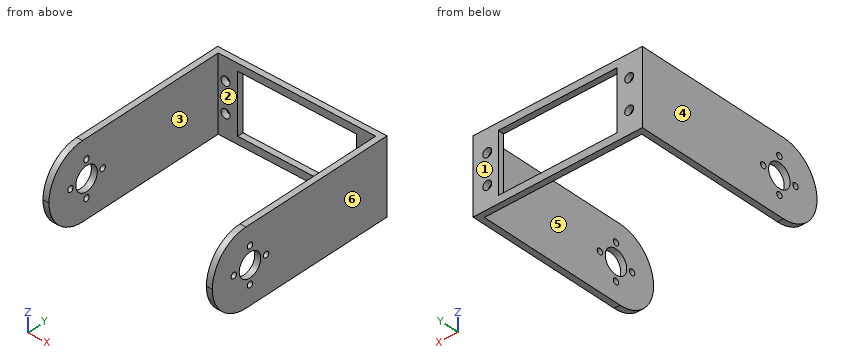
```python
from build123d import *

# Parameters (mm, degrees)
BOSS_EXTRUDE2_DEPTH = 25
SKETCH4_R           = 4
CUT_EXTRUDE1_DEPTH  = 108.5257706
SKETCH6_R           = 4
CUT_EXTRUDE2_DEPTH  = 78.032036302
CUT_EXTRUDE3_DEPTH  = 78.032036302
SKETCH9_R           = 1
CUT_EXTRUDE4_DEPTH  = 78.032036302
SKETCH10_R          = 1
CUT_EXTRUDE5_DEPTH  = 108.5257706
SKETCH11_R          = 1.5
SKETCH11_W          = 40
SKETCH11_H          = 20
CUT_EXTRUDE6_DEPTH  = 10


with BuildPart() as part:
    # Sketch3 → Boss-Extrude2 (new body)
    with BuildSketch(Plane.XY):
        Polygon((-79.925523148, 45.386502584), (-27.042967192, 45.386502584), (-24.925523148, 45.386502584), (-24.925523148, -19.613497416), (-26.925523148, -19.613497416), (-26.925523148, 43.389953837), (-79.925523148, 43.389953837), (-79.925523148, -19.613497416), (-81.925523148, -19.613497416), (-81.925523148, 45.386502584), align=None)
    extrude(amount=BOSS_EXTRUDE2_DEPTH)

    # Sketch4 → Cut-Extrude1 (cut, through all)
    with BuildSketch(Plane(origin=(0, 45.386502584, 0), x_dir=(1, 0, 0), z_dir=(0, 1, 0))):
        with Locations(Location((-54.925523148, -12.5, 0), (0, 0, 270))):
            Circle(SKETCH4_R)
    extrude(amount=-CUT_EXTRUDE1_DEPTH, mode=Mode.SUBTRACT)

    # Sketch6 → Cut-Extrude2 (cut, through all)
    with BuildSketch(Plane.ZY.offset(81.925523148)):
        with Locations(Location((12.5, -5.613497416, 0), (0, 0, 270))):
            Circle(SKETCH6_R)
    extrude(amount=-CUT_EXTRUDE2_DEPTH, mode=Mode.SUBTRACT)

    # Sketch8 → Cut-Extrude3 (cut, through all)
    with BuildSketch(Plane.ZY.offset(81.925523148)):
        with BuildLine():
            Line((0, -19.613497416), (12.5, -19.613497416))
            ThreePointArc((12.5, -19.613497416), (3.661165213, -15.952332159), (0, -7.113497352))
            Line((0, -7.113497352), (0, -19.613497416))
        make_face()
        with BuildLine():
            Line((12.5, -19.613497416), (25, -19.613497416))
            Line((25, -19.613497416), (25, -7.113497416))
            ThreePointArc((25, -7.113497416), (21.338834765, -15.952332181), (12.5, -19.613497416))
        make_face()
    extrude(amount=-CUT_EXTRUDE3_DEPTH, mode=Mode.SUBTRACT)

    # Sketch9 → Cut-Extrude4 (cut, through all)
    with BuildSketch(Plane(origin=(-24.925523148, 0, 0), x_dir=(0, 0, -1), z_dir=(1, 0, 0))):
        with Locations(Location((-6.5, -5.613497416, 0), (0, 0, 90))):
            Circle(SKETCH9_R)
        with Locations(Location((-12.5, -11.613497416, 0), (0, 0, 90))):
            Circle(SKETCH9_R)
        with Locations(Location((-18.5, -5.613497416, 0), (0, 0, 90))):
            Circle(SKETCH9_R)
        with Locations(Location((-12.5, 0.386502584, 0), (0, 0, 90))):
            Circle(SKETCH9_R)
    extrude(amount=-CUT_EXTRUDE4_DEPTH, mode=Mode.SUBTRACT)

    # Sketch10 → Cut-Extrude5 (cut, through all)
    with BuildSketch(Plane(origin=(0, 45.386502584, 0), x_dir=(1, 0, 0), z_dir=(0, 1, 0))):
        with Locations(Location((-60.925523148, -12.154997531, 0), (0, 0, 270))):
            Circle(SKETCH10_R)
        with Locations(Location((-54.580522888, -6.49999994, 0), (0, 0, 270))):
            Circle(SKETCH10_R)
        with Locations(Location((-48.925525297, -12.845000201, 0), (0, 0, 270))):
            Circle(SKETCH10_R)
        with Locations(Location((-55.270525558, -18.499997791, 0), (0, 0, 270))):
            Circle(SKETCH10_R)
    extrude(amount=-CUT_EXTRUDE5_DEPTH, mode=Mode.SUBTRACT)

    # Sketch11 → Cut-Extrude6 (cut)
    with BuildSketch(Plane(origin=(0, 45.386502584, 0), x_dir=(1, 0, 0), z_dir=(0, 1, 0))):
        with Locations(Location((-77.486757697, -7.5, 0), (0, 0, 270))):
            Circle(SKETCH11_R)
        with Locations(Location((-77.486757697, -17.5, 0), (0, 0, 270))):
            Circle(SKETCH11_R)
        with Locations(Location((-29.732572802, -17.5, 0), (0, 0, 270))):
            Circle(SKETCH11_R)
        with Locations(Location((-29.732572802, -7.5, 0), (0, 0, 270))):
            Circle(SKETCH11_R)
        with Locations((-53.425523148, -12.535744512)):
            Rectangle(SKETCH11_W, SKETCH11_H)
    extrude(amount=-CUT_EXTRUDE6_DEPTH, mode=Mode.SUBTRACT)


solid = part.part
```
Geometry: final body of the model. Coordinates: model frame, mm. Face numbers are marked on the shaded views. A direction names the side the tool comes from. Coordinates: 2 decimals unless noted, no trailing zeros. Order: outer loops, then holes, each group sorted by start corner. A loop starts at its lowest first (then second) coordinate and runs counter-clockwise, first axis right, second up. Notation, with made-up numbers: (69, -27) -> (107, -27) arc R18 ccw to (107, -8) -> close; hole circle Ø7 at (-24.5, 51.25). An arc over 180 degrees is marked (long way). Use CSV: the item, a comma, the result in double quotes.
1) Access query for the marked faces 5 and 6. Directions: +Z, -Z, +X, -X, +Y, -Y. A direction counts if a zero-diameter tool reaches every point of the face in a straight line with its end or side. Return the directions, or none.
Findings:
face 5,"+Z, -Z, -Y"
face 6,"+Z, -Z, +X, +Y, -Y"
2) Line query: line 1 (X direction, y = 44.55, z = 17.5); line 2 (X direction, y = 29, z = 8.75); line 3 (Y direction, x = -29.5, z = 2.75). Output: solid intervals per line, ascending.
Findings:
line 1,"x = -81.93 to -78.99, -75.99 to -73.43, -33.43 to -31.23, -28.23 to -24.93"
line 2,"x = -81.93 to -79.93, -26.93 to -24.93"
line 3,"y = 43.39 to 45.39"
3) Section A-A on x = -65.5. Output: boundary loops of the cut face in (y, z), then the cut area to 3 significant figures.
Findings:
outline,"(43.39, 0) -> (45.39, 0) -> (45.39, 2.54) -> (43.39, 2.54) -> close; (43.39, 22.54) -> (45.39, 22.54) -> (45.39, 25) -> (43.39, 25) -> close"
area,"9.98 mm^2"
4) Mould query, pull axis X, two halves, no side actions, for the marked faces 1, 2, 3 and 4. Classes: +X half, -X half, draft (parallel to the pull), parting line (faces both ways), or undercut.
Findings:
face 1,"draft"
face 2,"undercut"
face 3,"undercut"
face 4,"-X half"
5) Section B-B on y = 17.5. Output: boundary loops of the cut face in (x, z).
Findings:
outline,"(-81.93, 0) -> (-79.93, 0) -> (-79.93, 25) -> (-81.93, 25) -> close; (-26.93, 0) -> (-24.93, 0) -> (-24.93, 25) -> (-26.93, 25) -> close"
6) Pin query (flat end, axial travel): pin 1 Ø9 at (y, z) = (-5.61, 12.5) entering from -X; pin 2 Ø5 at (x, z) = (-49.5, 22) entering from -Y. Return the tip coordinate at first contact, or that it passes through.
Findings:
pin 1,"stops at x = -81.93"
pin 2,"stops at y = 43.39"
7) Section C-C on z = 15. Output: boundary loops of the cut face in (x, y).
Findings:
outline,"(-81.93, -19.36) -> (-79.93, -19.36) -> (-79.93, -8.74) -> (-81.93, -8.74) -> close; (-81.93, -2.49) -> (-79.93, -2.49) -> (-79.93, 43.39) -> (-73.43, 43.39) -> (-73.43, 45.39) -> (-81.93, 45.39) -> close; (-33.43, 43.39) -> (-26.93, 43.39) -> (-26.93, -2.49) -> (-24.93, -2.49) -> (-24.93, 45.39) -> (-33.43, 45.39) -> close; (-26.93, -19.36) -> (-24.93, -19.36) -> (-24.93, -8.74) -> (-26.93, -8.74) -> close"
